```python
from build123d import *

# Parameters (mm, degrees)
BOSS_EXTRUDE1_DEPTH       = 25.4
SKETCH2_W                 = 16.51
SKETCH2_H                 = 1.964574829
SKETCH2_H_2               = 1.210425171
CUT_EXTRUDE1_DEPTH        = 16.002
CUT_EXTRUDE2_DEPTH        = 4.445
CUT_EXTRUDE3_DEPTH        = 2.54
FILLET1_R                 = 12.7
F_2_CLEARANCE_HOLE1_D     = 2.4384
F_2_CLEARANCE_HOLE1_DEPTH = 25.4
F_2_CLEARANCE_HOLE1_TIP   = 0.732569267
F_6_32_TAPPED_HOLE1_D     = 2.7051
F_6_32_TAPPED_HOLE1_DEPTH = 9.398
F_6_32_TAPPED_HOLE1_TIP   = 0.81269403
CUT_EXTRUDE4_REACH        = 70.674


with BuildPart() as part:
    # Sketch1 → Boss-Extrude1 (new body)
    with BuildSketch(Plane.XY):
        Polygon((-22.352, -53.975), (-16.002, -53.975), (-16.002, -3.175), (0, -3.175), (0, 0), (25.654, 0), (25.654, 4.445), (-22.352, 4.445), align=None)
    extrude(amount=BOSS_EXTRUDE1_DEPTH)

    # Sketch2 → Cut-Extrude1 (cut)
    with BuildSketch(Plane(origin=(0, 0, 0), x_dir=(0, 0, -1), z_dir=(1, 0, 0))):
        with Locations((-12.7, -0.982287415)):
            Rectangle(SKETCH2_W, SKETCH2_H)
        with Locations((-12.7, -2.569787415)):
            Rectangle(SKETCH2_W, SKETCH2_H_2)
    extrude(amount=-CUT_EXTRUDE1_DEPTH, mode=Mode.SUBTRACT)

    # Sketch3 → Cut-Extrude2 (cut)
    with BuildSketch(Plane.XZ):
        with BuildLine():
            Line((-7.502, 14.351), (11.5, 14.351))
            ThreePointArc((11.5, 14.351), (13.151, 12.7), (11.5, 11.049))
            Line((11.5, 11.049), (-7.502, 11.049))
            ThreePointArc((-7.502, 11.049), (-9.153, 12.7), (-7.502, 14.351))
        make_face()
    extrude(amount=-CUT_EXTRUDE2_DEPTH, mode=Mode.SUBTRACT)

    # Sketch4 → Cut-Extrude3 (cut)
    with BuildSketch(Plane.XZ):
        with BuildLine():
            Line((-7.502, 16.51), (11.5, 16.51))
            ThreePointArc((11.5, 16.51), (15.31, 12.7), (11.5, 8.89))
            Line((11.5, 8.89), (-7.502, 8.89))
            ThreePointArc((-7.502, 8.89), (-11.312, 12.7), (-7.502, 16.51))
        make_face()
    extrude(amount=-CUT_EXTRUDE3_DEPTH, mode=Mode.SUBTRACT)

    # Fillet1
    fillet1_edges = [part.edges().sort_by_distance(p)[0] for p in [
        (25.654, 2.2225, 0),
        (25.654, 2.2225, 25.4),
    ]]
    fillet(fillet1_edges, radius=FILLET1_R - 0.0001)  # a hair under: the kernel refuses the full size

    # #2 Clearance Hole1
    with Locations(Plane(origin=(0, 4.445, 0), x_dir=(1, 0, 0), z_dir=(0, 1, 0))):
        with Locations((-7.002, -18.16), (-7.002, -7.24)):
            Hole(F_2_CLEARANCE_HOLE1_D / 2, depth=F_2_CLEARANCE_HOLE1_DEPTH)
            with Locations((0, 0, -(F_2_CLEARANCE_HOLE1_DEPTH + F_2_CLEARANCE_HOLE1_TIP / 2))):  # 118° drill point
                Cone(0, F_2_CLEARANCE_HOLE1_D / 2, F_2_CLEARANCE_HOLE1_TIP, mode=Mode.SUBTRACT)

    # #6-32 Tapped Hole1
    with Locations(Plane.ZY.offset(22.352)):
        with Locations((6.35, -9.525), (19.05, -9.525), (6.35, -47.625), (19.05, -47.625)):
            Hole(F_6_32_TAPPED_HOLE1_D / 2, depth=F_6_32_TAPPED_HOLE1_DEPTH)
            with Locations((0, 0, -(F_6_32_TAPPED_HOLE1_DEPTH + F_6_32_TAPPED_HOLE1_TIP / 2))):  # 118° drill point
                Cone(0, F_6_32_TAPPED_HOLE1_D / 2, F_6_32_TAPPED_HOLE1_TIP, mode=Mode.SUBTRACT)

    # Cut-Extrude4: up to this face of the body (flat: up to its plane)
    cut_extrude4_end = Plane(part.part.faces().sort_by_distance((-8.001, -3.175, 23.1775))[0])
    # Sketch10 → Cut-Extrude4 (cut, up to the picked face)
    with BuildSketch(Plane(origin=(0, 4.445, 0), x_dir=(1, 0, 0), z_dir=(0, 1, 0)), mode=Mode.PRIVATE) as cut_extrude4_sk1:
        with BuildLine():
            Line((-7.502, -25.4), (30.598, -25.4))
            Line((30.598, -25.4), (30.598, 0))
            Line((30.598, 0), (-7.502, 0))
            ThreePointArc((-7.502, 0), (5.198, -12.7), (-7.502, -25.4))
        make_face()
    cut_extrude4_tool1 = split(extrude(cut_extrude4_sk1.sketch, amount=-CUT_EXTRUDE4_REACH, mode=Mode.PRIVATE), bisect_by=cut_extrude4_end, keep=Keep.BOTH, mode=Mode.PRIVATE)
    add(cut_extrude4_tool1.solids().sort_by(Axis((16.392438, 4.445, 12.7), (0, -1, 0)))[0], mode=Mode.SUBTRACT)


solid = part.part
```
Geometry check sheet. Reference: the model listing, model coordinates, mm. A direction names the side the tool comes from. Give positions to 0.01 mm unless a question says otherwise; leave off trailing zeros. Order: outer loops, then holes, each group sorted by start corner. A loop starts at its lowest first (then second) coordinate and runs counter-clockwise, first axis right, second up.
1. Section check A-A, the plane x = 1.5. Enter the section's corners in (y, z) (3 decimals), and give its area (3 significant figures).
2. Section check D-D, the plane y = -7. Enter the section's corners in (x, z).
3. Gauge pin test, flat ends, axial feed: pin 1 Ø3 at (y, z) = (-9.525, 19.05) entering from +X; pin 2 Ø8.5 at (x, z) = (-2.5, 12.5) entering from -Y; pin 3 Ø1.5 at (x, y) = (1.5, 4) entering from +Z. Record the tip position at first contact, or that the pin passes through.
4. Section check C-C, the plane x = -6.75. Enter the section's corners in (y, z) (3 decimals).
5. Section check B-B, the plane z = 12.7. Enter the section's corners in (x, y) (3 decimals), and give its area (3 significant figures).
6. Access from +Z, -Z, +X, -X, +Y, -Y to the whole of each face (thin tool, end or side, straight path). Record for faces 5 (the face through (-18, -24, 0)), 6 (the face through (-8, -3.175, 2)), 7 (the face through (-2, 1, 16.51)).
7. Release check for a two-part mould opening along Y. For faces 1 (the face through (-8, -2, 4.445)), 2 (the face through (-19.13, -9.12, 17.76)), 3 (the face through (-19, -53.975, 13)), 4 (the face through (-19.133, -8.184, 6.526)) record: pulls with the +Y half, pulls with the -Y half, needs draft (parallel to the pull), parting line crosses it, or undercut.
8. Thickness scan on L1, parallel to Y at x = -19.25, z = 6.35 (3 decimals); L2, parallel to X at y = -49.5, z = 5.75; L3, parallel to Y at x = -12.75, z = 20 (3 decimals). Record the ranges inside material, lowest first.
Values follow:
1. outline: (0, 3.742) - (4.445, 3.742) - (4.445, 11.049) - (2.54, 11.049) - (2.54, 8.89) - (0, 8.89) - close; (0, 16.51) - (2.54, 16.51) - (2.54, 14.351) - (4.445, 14.351) - (4.445, 21.658) - (0, 21.658) - close
1. area: 54.0 mm2
2. outline: (-22.35, 0) - (-16, 0) - (-16, 25.4) - (-22.35, 25.4) - close
3. pin 1: stops at x = -16
3. pin 2: stops at y = 0
3. pin 3: stops at z = 22.35
4. outline: (-3.175, 0.022) - (4.445, 0.022) - (4.445, 6.047) - (0, 6.047) - (0, 4.445) - (-3.175, 4.445) - close; (-3.175, 20.955) - (0, 20.955) - (0, 19.353) - (4.445, 19.353) - (4.445, 25.378) - (-3.175, 25.378) - close; (0, 8.433) - (4.445, 8.433) - (4.445, 11.049) - (2.54, 11.049) - (2.54, 8.89) - (0, 8.89) - close; (0, 16.51) - (2.54, 16.51) - (2.54, 14.351) - (4.445, 14.351) - (4.445, 16.967) - (0, 16.967) - close
5. outline: (-22.352, -53.975) - (-16.002, -53.975) - (-16.002, 0) - (-11.312, 0) - (-11.312, 2.54) - (-9.153, 2.54) - (-9.153, 4.445) - (-22.352, 4.445) - close
5. area: 396 mm2
6. face 5: -Z, +X, -X, +Y, -Y
6. face 6: +Z, -Z, +X, -Y
6. face 7: +X, -Y
7. face 1: needs draft
7. face 2: undercut
7. face 3: pulls with the -Y half
7. face 4: undercut
8. L1: y = -53.975 to -48.978, -46.272 to -10.878, -8.172 to 4.445
8. L2: x = -22.35 to -16
8. L3: y = 0 to 4.445
